Design review of the part built by this model. Coordinates are the model's own, in mm. Face numbers are marked on the shaded views. Round coordinates to 2 decimals unless told otherwise and drop trailing zeros. Write each loop counter-clockwise with the first axis right and the second up, starting at its lowest first coordinate (ties: lowest second). Pieces come first, ordered by that corner, then holes. Notation, with made-up numbers: M 54.5,78 L 109.5,78 A9 cw 109.5,89 Z; hole C 36.25,66.25 d7. An arc over 180 degrees is marked long. One line per question, with ' | ' between items. Start each with the question number.
Item 1: Add section C-C, the plane y = -18.5. State the section outline as (x, z) points.
Item 2: Add section B-B, the plane x = 69. State the section outline as (y, z) points, and give its area (3 significant figures).
Item 3: Insertion check: pin 1 Ø23 at (x, y) = (-33.5, -20.5) entering from +Z; pin 2 Ø8 at (x, y) = (-73.5, 8.5) entering from -Z; pin 3 Ø4 at (x, y) = (-10.93, 7.13) entering from -Z. Each pin has a flat end and moves straight along its axis. Give the tip position at first contact, or say it passes through.
Item 4: Add section A-A, the plane z = 5.25. State the section outline as (x, y) points.
Item 5: For L1, parallel to Y at x = -4.5, z = 6; L2, parallel to X at y = -30.5, z = 3.5; L3, parallel to X at y = 8.5, z = 3.25, list the stretches that pass through material, from the lowest coordinate up.
Item 6: Draft analysis for pull direction Y (two halves, no side actions). For the marked faces 1 and 2, state which applies: released by +Y, released by -Y, zero draft, split by the parting line, or undercut.
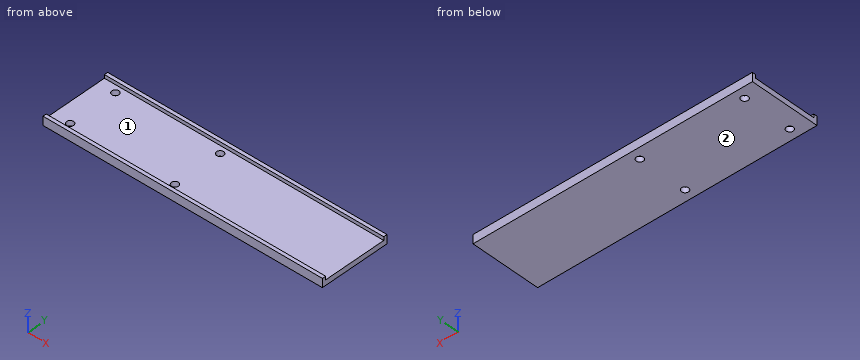
```python
from build123d import *

# Parameters (mm, degrees)
F0_W     = 203.2
F0_H     = 50.8
F1_DEPTH = 3.81
F2_W     = 203.2
F2_H     = 2.54
F3_DEPTH = 2.54
F4_R     = 2.54
F5_DEPTH = 3.81


with BuildPart() as f1:
    # F0 (on Top) → F1 (new body)
    with BuildSketch(Plane.XY):
        with Locations((1.766223, -10.64699)):
            Rectangle(F0_W, F0_H)
    extrude(amount=F1_DEPTH)

    # F2 (on face) → F3 (join)
    with BuildSketch(Plane.XY.offset(3.81)):
        with Locations((1.766223, 13.48301)):
            Rectangle(F2_W, F2_H)
        with Locations((1.766223, -34.77699)):
            Rectangle(F2_W, F2_H)
    extrude(amount=F3_DEPTH)

    # F4 (on face) → F5 (cut)
    with BuildSketch(Plane.XY.offset(3.81)):
        with Locations((-87.133777, 7.13301)):
            Circle(F4_R)
        with Locations((-87.133777, -28.42699)):
            Circle(F4_R)
        with Locations((-10.933777, 7.13301)):
            Circle(F4_R)
        with Locations((-10.933777, -28.42699)):
            Circle(F4_R)
    extrude(amount=-F5_DEPTH, mode=Mode.SUBTRACT)


solid = f1.part
```
Computed values:
1) outline: M -99.83,0 L 103.37,0 L 103.37,3.81 L -99.83,3.81 Z
2) outline: M -36.05,0 L 14.75,0 L 14.75,6.35 L 12.21,6.35 L 12.21,3.81 L -33.51,3.81 L -33.51,6.35 L -36.05,6.35 Z | area: 206 mm^2
3) pin 1: stops at z = 3.81 | pin 2: stops at z = 0 | pin 3: passes through
4) outline: M -99.83,-36.05 L 103.37,-36.05 L 103.37,-33.51 L -99.83,-33.51 Z; M -99.83,12.21 L 103.37,12.21 L 103.37,14.75 L -99.83,14.75 Z
5) L1: y = -36.05 to -33.51, 12.21 to 14.75 | L2: x = -99.83 to -88.6, -85.67 to -12.4, -9.47 to 103.37 | L3: x = -99.83 to -89.27, -84.99 to -13.07, -8.79 to 103.37
6) face 1: undercut | face 2: zero draft
